from build123d import *

# Parameters (mm, degrees)
SKETCH1_W          = 19.05
SKETCH1_H          = 19.05
SKETCH1_R          = 4.7625
BASE_EXTRUDE_DEPTH = 9.525
SKETCH3_R          = 4.7625
CUT_EXTRUDE1_DEPTH = 24.3313898
SCALE1_SCALE       = 0.8


with BuildPart() as part:
    # Sketch1 → Base-Extrude (new, symmetric)
    with BuildSketch(Plane.XY):
        Rectangle(SKETCH1_W, SKETCH1_H)
        with Locations(Location((0, 0, 0), (0, 0, 180))):
            Circle(SKETCH1_R, mode=Mode.SUBTRACT)
    extrude(amount=BASE_EXTRUDE_DEPTH, both=True)

    # Sketch3 → Cut-Extrude1 (cut, through all)
    with BuildSketch(Plane(origin=(9.525, 0, 0), x_dir=(0, 0, -1), z_dir=(1, 0, 0))):
        Circle(SKETCH3_R)
    extrude(amount=-CUT_EXTRUDE1_DEPTH, mode=Mode.SUBTRACT)


with BuildPart() as part_1:
    # Scale1: scaled about (0, 0, 0)
    add(part.part.scale(SCALE1_SCALE))


solid = part_1.part
Could you check a few things on this model? Use its own coordinates, in mm. Give positions to 0.01 mm unless a question says otherwise; leave off trailing zeros. Order: outer loops, then holes, each group sorted by start corner. A loop starts at its lowest first (then second) coordinate and runs counter-clockwise, first axis right, second up.
1. Thinking about a two-plate mould opening in Y: for faces 1 (the cylindrical face through (4.71, 3.21, -2.05)), 2 (the flat face through (0, 7.62, 0)), 3 (the flat face through (-3, 3, 7.62)), which applies, +Y half, -Y half, draft (parallel to the pull), parting line (faces both ways), or undercut?
Answers below:
face 1: undercut
face 2: +Y half
face 3: draft
2. Suppose I cut it at C-C (z = -1.5). Write out the boundary of the cut face in (x, y), plus the area to 3 significant figures.
Answers below:
outline: (-7.62, -7.62) - (7.62, -7.62) - (7.62, -3.5) - (1.5, -3.5) arc R3.81 cw to (-1.5, -3.5) - (-7.62, -3.5) - close; (-7.62, 3.5) - (-1.5, 3.5) arc R3.81 cw to (1.5, 3.5) - (7.62, 3.5) - (7.62, 7.62) - (-7.62, 7.62) - close
area: 124 mm2
3. Suppose I cut it at D-D (x = -0.75). Write out the boundary of the cut face in (y, z), plus the area to 3 significant figures.
Answers below:
outline: (-7.62, -7.62) - (-3.74, -7.62) - (-3.74, -0.75) arc R3.81 cw to (-3.74, 0.75) - (-3.74, 7.62) - (-7.62, 7.62) - close; (3.74, -7.62) - (7.62, -7.62) - (7.62, 7.62) - (3.74, 7.62) - (3.74, 0.75) arc R3.81 cw to (3.74, -0.75) - close
area: 118 mm2
4. Suppose I cut it at B-B (x = -5). Write out the boundary of the cut face in (y, z).
Answers below:
outline: (-7.62, -7.62) - (7.62, -7.62) - (7.62, 7.62) - (-7.62, 7.62) - close; hole circle Ø7.62 at (0, 0)
5. Suppose I cut it at A-A (y = 0). Write out the boundary of the cut face in (x, z).
Answers below:
outline: (-7.62, -7.62) - (-3.81, -7.62) - (-3.81, -3.81) - (-7.62, -3.81) - close; (-7.62, 3.81) - (-3.81, 3.81) - (-3.81, 7.62) - (-7.62, 7.62) - close; (3.81, -7.62) - (7.62, -7.62) - (7.62, -3.81) - (3.81, -3.81) - close; (3.81, 3.81) - (7.62, 3.81) - (7.62, 7.62) - (3.81, 7.62) - close
6. I need wall thicknesses on L1, parallel to Y at x = 0, z = 5; L2, parallel to X at y = 3, z = -4.75; L3, parallel to Z at x = 7.25, y = -2. Which ranges of each line are inside material? Lowest first, please.
Answers below:
L1: y = -7.62 to -3.81, 3.81 to 7.62
L2: x = -7.62 to -2.35, 2.35 to 7.62
L3: z = -7.62 to -3.24, 3.24 to 7.62
7. For pin 1 (6 mm diameter, centred on x = 0, y = 0, fed in from -Z), with a flat end and sliding along its axis, tell me the tip position at first contact or that it passes through.
Answers below:
pin 1: passes through
